Could you check a few things on this model? Use its own coordinates, in mm. A direction names the side the tool comes from. Give positions to 0.01 mm unless a question says otherwise; leave off trailing zeros. Order: outer loops, then holes, each group sorted by start corner. A loop starts at its lowest first (then second) coordinate and runs counter-clockwise, first axis right, second up.
(1) Will these pins go through, and if not, where does the flat tip stop? pin 1 (6 mm diameter, centred on x = -7, z = -1, fed in from -Y); pin 2 (1 mm diameter, centred on x = 3.5, y = 0.5, fed in from -Z).
(2) On a 3-axis mill with a long thin cutter (end or side, diameter ignored), from which of +Z, -Z, +X, -X, +Y, -Y can I reach the whole of each face in a straight line? I mean faces 1 (the cylindrical face through (-5.37, 1.48, -1.19)), 2 (the flat face through (7, 1, -4.3)). Say none if no direction works.
(3) Imagine slicing it at C-C, the plane y = 2.55. Write out the boundary of the cut face in (x, z).
(4) If I drill on probe 1 along Y at (x, z) = (4, -7.75); probe 2 along X at (y, z) = (2.1, 0); probe 3 along X at (y, z) = (2.3, 5), over which ranges is the centre line in solid material (lowest first)?
(5) If we mould it in two halves opening along Y, with no side actions, what happens to faces 3 (the flat face through (-7, 2, -4.3)), 4 (the cylindrical face through (-5.78, 2.49, -7.54)), 5 (the flat face through (-4, 3, 4))? For each: released by +Y, released by -Y, zero draft, split by the parting line, or undercut.
from build123d import *

# Parameters (mm, degrees)
SKETCH1_R           = 7.5
SKETCH1_R_2         = 5.5
BOSS_EXTRUDE1_DEPTH = 3
BOSS_EXTRUDE2_START = -1
SKETCH2_R           = 9.5
SKETCH2_R_2         = 7.5
BOSS_EXTRUDE2_DEPTH = 1
SKETCH3_R           = 9.5
SKETCH3_R_2         = 7.5
BOSS_EXTRUDE3_DEPTH = 1
FILLET1_R           = 0.5


with BuildPart() as part:
    # Sketch1 → Boss-Extrude1 (new body)
    with BuildSketch(Plane(origin=(0, 0, 0), x_dir=(1, 0, 0), z_dir=(0, 1, 0))):
        with Locations(Location((0, 0, 0), (0, 0, 270))):
            Circle(SKETCH1_R)
        with Locations(Location((0, 0, 0), (0, 0, 270))):
            Circle(SKETCH1_R_2, mode=Mode.SUBTRACT)
    extrude(amount=BOSS_EXTRUDE1_DEPTH)

    # Sketch2 → Boss-Extrude2 (add)
    with BuildSketch(Plane(origin=(0, 3, 0), x_dir=(1, 0, 0), z_dir=(0, 1, 0)).offset(BOSS_EXTRUDE2_START)):
        with Locations(Location((0, 0, 0), (0, 0, 270))):
            Circle(SKETCH2_R)
        with Locations(Location((0, 0, 0), (0, 0, 270))):
            Circle(SKETCH2_R_2, mode=Mode.SUBTRACT)
    extrude(amount=BOSS_EXTRUDE2_DEPTH)

    # Sketch3 → Boss-Extrude3 (add)
    with BuildSketch(Plane.XZ):
        with Locations(Location((0, 0, 0), (0, 0, 90))):
            Circle(SKETCH3_R)
        with Locations(Location((0, 0, 0), (0, 0, 270))):
            Circle(SKETCH3_R_2, mode=Mode.SUBTRACT)
    extrude(amount=-BOSS_EXTRUDE3_DEPTH)

    # Fillet1
    fillet1_edges = [part.edges().sort_by_distance(p)[0] for p in [
        (0, 2, -7.5),
        (0, 1, -7.5),
    ]]
    fillet(fillet1_edges, radius=FILLET1_R - 0.0001)  # a hair under: the kernel refuses the full size


solid = part.part
Answer block:
1. pin 1: stops at y = 0
1. pin 2: stops at z = -9.01
2. face 1: +Y, -Y
2. face 2: none
3. outline: circle Ø19 at (0, 0); hole circle Ø11 at (0, 0)
4. probe 1: y = 0 to 1, 2 to 3
4. probe 2: x = -9.5 to -5.5, 5.5 to 9.5
4. probe 3: x = -8.08 to -2.29, 2.29 to 8.08
5. face 3: undercut
5. face 4: zero draft
5. face 5: released by +Y
